Geometry check sheet. Reference: the model listing, model coordinates, mm. A direction names the side the tool comes from. Round coordinates to 2 decimals unless told otherwise and drop trailing zeros. Loops run counter-clockwise (first coordinate to the right, second up) from the corner with the lowest first, then second, coordinate; pieces in that order, holes last. Notation, with made-up numbers: M 60.5,-21.75 L 103.5,-21.75 A20 cw 103.5,-8.75 Z; hole C 80.25,72 d9. An arc over 180 degrees is marked long. Write item = value, one per line.
from build123d import *

# Parameters (mm, degrees)
BOSS_EXTRUDE1_DEPTH = 1.5875
FILLET1_R           = 1.27
FILLET2_R           = 0.254
FILLET3_R           = 2.794


with BuildPart() as part:
    # Sketch1 → Boss-Extrude1 (new body)
    with BuildSketch(Plane.XY):
        Polygon((5.651886258, 2.848562209), (34.979186258, 2.848562209), (34.979186258, 6.175962209), (32.947186258, 6.175962209), (32.947186258, 5.388562209), (8.191886258, 5.388562209), (8.191886258, 11.484562209), (34.979186258, 11.484562209), (34.979186258, 14.024562209), (5.651886258, 14.024562209), align=None)
    extrude(amount=BOSS_EXTRUDE1_DEPTH)

    # Fillet1
    fillet1_edges = [part.edges().sort_by_distance(p)[0] for p in [
        (5.651886258, 14.024562209, 0.79375),
        (34.979186258, 14.024562209, 0.79375),
        (34.979186258, 11.484562209, 0.79375),
        (34.979186258, 6.175962209, 0.79375),
        (34.979186258, 2.848562209, 0.79375),
        (5.651886258, 2.848562209, 0.79375),
    ]]
    fillet(fillet1_edges, radius=FILLET1_R - 0.0001)  # a hair under: the kernel refuses the full size

    # Fillet2
    fillet2_edges = [part.edges().sort_by_distance(p)[0] for p in [
        (32.947186258, 5.388562209, 0.79375),
        (32.947186258, 6.175962209, 0.79375),
    ]]
    fillet(fillet2_edges, radius=FILLET2_R)

    # Fillet3
    fillet3_edges = [part.edges().sort_by_distance(p)[0] for p in [
        (8.191886258, 11.484562209, 0.79375),
        (8.191886258, 5.388562209, 0.79375),
    ]]
    fillet(fillet3_edges, radius=FILLET3_R)


solid = part.part
(1) Sectioned sample at D-D on y = 9.5. Record the cut outline in (x, z), then the cut area to 3 significant figures.
Result set:
outline = M 5.65,0 L 8.31,0 L 8.31,1.59 L 5.65,1.59 Z
area = 4.22 mm2
(2) Release check for a two-part mould opening along Y. For faces 1 (the cylindrical face through (6.034, 3.211, 0.805)), 2 (the cylindrical face through (6.03, 13.66, 0.8)), 3 (the cylindrical face through (34.6, 11.85, 0.8)) record: released by +Y, released by -Y, zero draft, split by the parting line, or undercut.
Result set:
face_1 = released by -Y
face_2 = released by +Y
face_3 = undercut
(3) Sectioned sample at C-C on y = 11. Record the cut outline in (x, z).
Result set:
outline = M 5.65,0 L 9.41,0 L 9.41,1.59 L 5.65,1.59 Z
(4) Material ranges on line 1 along Y through (x, z) = (11.75, 0.45); line 2 along X through (y, z) = (8, 1.2); line 3 along X through (y, z) = (11.75, 0.55), recorded low to high. Write a range as from..to.
Result set:
line_1 = 2.85..5.39, 11.48..14.02
line_2 = 5.65..8.2
line_3 = 5.65..34.49
(5) Sectioned sample at A-A on x = 15. Record the cut outline in (y, z).
Result set:
outline = M 2.85,0 L 5.39,0 L 5.39,1.59 L 2.85,1.59 Z; M 11.48,0 L 14.02,0 L 14.02,1.59 L 11.48,1.59 Z
(6) Tool access check on faces 4 (the cylindrical face through (8.989, 10.644, 0.805)), 5 (the cylindrical face through (34.597, 3.211, 0.805)), 6 (the flat face through (22, 5.389, 1)). Record the directions out of +Z, -Z, +X, -X, +Y, -Y that give a thin tool (end or side, any length) a straight path to the whole face; none if there is none.
Result set:
face_4 = +Z, -Z, +X
face_5 = +Z, -Z, +X, -Y
face_6 = +Z, -Z
